Autodesk Inventor part; units mm, degrees
ref_plane "YZ Plane" through (0, 0, 0) normal (1, 0, 0) x (0, 1, 0)
ref_plane "XZ Plane" through (0, 0, 0) normal (0, 1, 0) x (-1, 0, 0)
ref_plane "XY Plane" through (0, 0, 0) normal (0, 0, 1) x (1, 0, 0)
sketch "Sketch1" plane through (0, 0, 0) normal (0, 1, 0) x (-1, 0, 0)
  arc A0 (-2.1359, -2.7727) -> (-2.1359, 2.7727) centre (0, 0) ccw
  line L0 (3.4641, 0.5) -> (-2.1359, 0.5)
  line L1 (-2.1359, 0.5) -> (-2.1359, -2.7727)
  line L2 (-2.1359, 0.5) -> (-2.1359, 2.7727)
  line L3 (-3.6359, 3.4322) -> (-3.6359, 0.5)
  line L4 (-3.6359, 0.5) -> (-3.6359, -3.4322)
  arc A1 (-3.6359, -3.4322) -> (-3.6359, 3.4322) centre (0, 0) ccw
  dimension "d0" = 7
  dimension "d1" = 5.6
  dimension "d2" = 3
  dimension "d3" = 1.5
extrude "Extrusion1" add sketch "Sketch1" along normal blind 21
sketch "Sketch2" plane through (0, 21, 0) normal (0, 1, 0) x (1, 0, 0)
  line L0 (3.6359, -3.4322) -> (3.6359, 3.4322)
  arc A0 (3.6359, 3.4322) -> (3.6359, -3.4322) centre (0, 0) ccw
  line L1 (2.1359, 2.7727) -> (2.1359, -2.7727)
  arc A1 (2.1359, 2.7727) -> (2.1359, -2.7727) centre (0, 0) ccw
extrude "Extrusion2" add sketch "Sketch2" along normal blind 2.5 contours A0 L0 | L1 A1
sketch "Sketch4" plane through (0, 23.5, 0) normal (0, 1, 0) x (1, 0, 0)
  arc A0 (3.6359, 3.4322) -> (3.6359, -3.4322) centre (0, 0) ccw
  line L0 (3.6359, -3.4322) -> (3.6359, 3.4322)
  circle A1 centre (0, 0) radius 5
  line L1 (0, -5) -> (-37.5, -5)
  line L2 (-40, -2.5) -> (-40, 2.5)
  line L3 (-37.5, 5) -> (0, 5)
  arc A2 (-40, -2.5) -> (-37.5, -5) centre (-37.5, -2.5) ccw
  arc A3 (-37.5, 5) -> (-40, 2.5) centre (-37.5, 2.5) ccw
  line L4 (-35.0895, 0) -> (-28.9105, 0) construction
  line L5 (-35.0895, -2) -> (-28.9105, -2)
  line L6 (-28.9105, 2) -> (-35.0895, 2)
  arc A4 (-35.0895, 2) -> (-35.0895, -2) centre (-35.0895, 0) ccw
  arc A5 (-28.9105, -2) -> (-28.9105, 2) centre (-28.9105, 0) ccw
  line L7 (-22.9105, 5) -> (-22.9105, -5)
  line L8 (-10.7314, 0) -> (-16.9105, 0) construction
  line L9 (-10.7314, -2) -> (-16.9105, -2)
  line L10 (-16.9105, 2) -> (-10.7314, 2)
  arc A6 (-10.7314, -2) -> (-10.7314, 2) centre (-10.7314, 0) ccw
  arc A7 (-16.9105, 2) -> (-16.9105, -2) centre (-16.9105, 0) ccw
  point P0 (-40, -5)
  point P1 (-32, 0)
  point P2 (-40, 0)
  point P3 (-26.9105, 0)
  point P4 (-8.321, -2.5)
  point P5 (-8.321, 2.5)
  point P6 (-13.821, 0)
  point P7 (-18.9105, 0)
  point P8 (3.6359, -3.4322)
  point P9 (3.6359, 3.4322)
  dimension "d28" = 40
  dimension "d29" = 2.5
  dimension "d30" = 4
  dimension "d31" = 8
  dimension "d32" = 4
  dimension "d33" = 26.5464
extrude "Extrusion4" add sketch "Sketch4" along normal blind 4
properties part number "Sensor_Connect_Knob_Brake"
Geometry check sheet. Reference: the model listing, model coordinates, mm. A direction names the side the tool comes from. Give positions to 0.01 mm unless a question says otherwise; leave off trailing zeros. Write each loop counter-clockwise with the first axis right and the second up, starting at its lowest first coordinate (ties: lowest second). Pieces come first, ordered by that corner, then holes.
1) Material ranges on L1, parallel to X at y = 16.25, z = 0; L2, parallel to Z at x = 0, y = 7.75; L3, parallel to X at y = 25.25, z = -1.75, recorded low to high.
2) Section check B-B, the plane y = 20. Record the boundary of the cut face in (x, z).
3) Access from +Z, -Z, +X, -X, +Y, -Y to the whole of each face (thin tool, end or side, straight path). Record for faces 4 (the flat face through (-18, 27.5, 2)), 5 (the flat face through (3.636, 12, 0)), 6 (the flat face through (2.3, 0, 0.1)), 7 (the cylindrical face through (-3.5, 10.4, 0.1)), 8 (the cylindrical face through (-18.91, 25.47, 0.04)).
4) Release check for a two-part mould opening along Z. For faces 1 (the flat face through (-32, 25, -2)), 2 (the flat face through (-18, 25, 5)), 3 (the cylindrical face through (5, 25, 0)) record: pulls with the +Z half, pulls with the -Z half, needs draft (parallel to the pull), parting line crosses it, or undercut.
5) Section check A-A, the plane z = 0. Record the boundary of the cut face in (x, y).
6) Gauge pin test, flat ends, axial feed: pin 1 (3 mm diameter, centred on x = -14, z = 2, fed in from -Y); pin 2 (3 mm diameter, centred on y = 16.5, z = -2.5, fed in from -X); pin 3 (5 mm diameter, centred on y = 18, z = 2.5, fed in from -X); pin 4 (12 mm diameter, centred on x = -25.5, y = 13, fed in from +Z). Record the tip position at first contact, or that the pin passes through.
Computed:
1. L1: x = -5 to -3.5, 2.14 to 3.64
1. L2: z = -5 to -3.5, 3.5 to 5
1. L3: x = -40 to -36.06, -27.94 to -17.88, -9.76 to 4.68
2. outline: (3.64, -3.43) - (3.64, 3.43) arc R5 ccw (long way) to start; hole (2.14, -2.77) - (2.14, 2.77) arc R3.5 ccw (long way) to start
3. face 4: +Z, -Z, +X, -X, +Y
3. face 5: +Z, -Z, +X, -Y
3. face 6: +Z, -Z, +X, -X, -Y
3. face 7: -Y
3. face 8: +Y, -Y
4. face 1: undercut
4. face 2: pulls with the +Z half
4. face 3: parting line crosses it
5. outline: (-40, 23.5) - (-37.09, 23.5) - (-37.09, 27.5) - (-40, 27.5) - close; (-26.91, 23.5) - (-18.91, 23.5) - (-18.91, 27.5) - (-26.91, 27.5) - close; (-8.73, 23.5) - (-5, 23.5) - (-5, 0) - (-3.5, 0) - (-3.5, 21) - (2.14, 21) - (2.14, 0) - (3.64, 0) - (3.64, 23.5) - (5, 23.5) - (5, 27.5) - (-8.73, 27.5) - close
6. pin 1: stops at y = 23.5
6. pin 2: stops at x = -4.9
6. pin 3: stops at x = -5
6. pin 4: passes through
